Work out the finished part from the listing and answer in its coordinate system (mm). A direction names the side the tool comes from. Give positions to 0.01 mm unless a question says otherwise; leave off trailing zeros. Loops run counter-clockwise (first coordinate to the right, second up) from the corner with the lowest first, then second, coordinate; pieces in that order, holes last. Notation, with made-up numbers: M 6.5,50.5 L 20.5,50.5 A21 cw 20.5,86.5 Z; hole C 51,66 d10. An arc over 180 degrees is marked long. Answer in a Markdown table with one row per item. Add a question column.
from build123d import *

# Parameters (mm, degrees)
F0_R         = 38.1
F0_R_2       = 31.75
F1_DEPTH     = 26.924
F2_R         = 2.4528409794
F4_START     = -34.036
F3_W         = 36.8709713221
F3_H         = 33.7369362824
F4_DEPTH     = 4.826
F5_R         = 5.08
F6_W         = 26.7109713221
F6_H         = 23.5769362824
F7_DEPTH     = 4.826
F8_T1_DEPTH  = 26.7109713221
F8_T3_DEPTH  = 23.5769362824
F8_T6_ANGLE  = 90
F8_T8_ANGLE  = 90
F8_T10_ANGLE = 90
F8_T12_ANGLE = 90
F9_W         = 6.8778875601
F9_H         = 2.9623268638
F10_DEPTH    = 4.8006
F12_START    = 31.75
F11_W        = 2.54
F11_H        = 2.54
F12_DEPTH    = 7.874


# Not quite as in the source:
# - a fillet or chamfer that OpenCascade refuses, or shapes differently, is made with other operations: its cross-section is extruded or revolved along the edge and cut away or added


with BuildPart() as f1:
    # F0 (on Front) → F1 (new body)
    with BuildSketch(Plane.XZ):
        Circle(F0_R)
        Circle(F0_R_2, mode=Mode.SUBTRACT)
    extrude(amount=F1_DEPTH)

    # F2
    f2_edges = [f1.edges().sort_by_distance(p)[0] for p in [
        (-38.1, -26.924, 0),
        (-38.1, 0, 0),
    ]]
    fillet(f2_edges, radius=F2_R)

    # F3 (on Top) → F4 (join)
    with BuildSketch(Plane.XY.offset(F4_START)):
        with Locations((0.0921785831, -14.0109679196)):
            Rectangle(F3_W, F3_H)
    extrude(amount=-F4_DEPTH)

    # F5
    f5_edges = [f1.edges().sort_by_distance(p)[0] for p in [
        (-18.343307, 2.8575, -36.449),
        (18.527664, 2.8575, -36.449),
        (18.527664, -30.879436, -36.449),
        (-18.343307, -30.879436, -36.449),
    ]]
    fillet(f5_edges, radius=F5_R)

    # F6 (on face) → F7 (cut)
    with BuildSketch(Plane(origin=(0, 0, -38.862), x_dir=(1, 0, 0), z_dir=(0, 0, -1))):
        with Locations((0.0921785831, 14.0109679196)):
            Rectangle(F6_W, F6_H)
    extrude(amount=-F7_DEPTH, mode=Mode.SUBTRACT)

    # F8: fillet of radius 5.08 on 1 edges, made by hand

    # F8_s2 → F8_t1 (cut)
    with BuildSketch(Plane.YZ.offset(-13.2633070779)):
        with BuildLine():
            ThreePointArc((-30.8794360608, -34.036), (-29.3069384175, -37.4628096935), (-25.8057900345, -38.862))
            Line((-25.8057900345, -38.862), (-30.8794360608, -38.862))
            Line((-30.8794360608, -38.862), (-30.8794360608, -34.036))
        make_face()
        with BuildLine():
            ThreePointArc((2.8575002216, -34.036), (1.2850025783, -37.4628096935), (-2.2161458047, -38.862))
            Line((-2.2161458047, -38.862), (2.8575002216, -38.862))
            Line((2.8575002216, -38.862), (2.8575002216, -34.036))
        make_face()
    extrude(amount=F8_T1_DEPTH, mode=Mode.SUBTRACT)

    # F8_s4 → F8_t3 (cut)
    with BuildSketch(Plane.XZ.offset(2.2224997784)):
        with BuildLine():
            ThreePointArc((18.5276642442, -34.036), (16.9551666009, -37.4628096935), (13.4540182179, -38.862))
            Line((13.4540182179, -38.862), (18.5276642442, -38.862))
            Line((18.5276642442, -38.862), (18.5276642442, -34.036))
        make_face()
        with BuildLine():
            ThreePointArc((-18.3433070779, -34.036), (-16.7708094346, -37.4628096935), (-13.2696610516, -38.862))
            Line((-13.2696610516, -38.862), (-18.3433070779, -38.862))
            Line((-18.3433070779, -38.862), (-18.3433070779, -34.036))
        make_face()
    extrude(amount=F8_T3_DEPTH, mode=Mode.SUBTRACT)

    # F8_s5 → F8_t6 (revolve, cut)
    with BuildSketch(Plane.YZ.offset(-13.2633070779)):
        with BuildLine():
            ThreePointArc((-30.8794360608, -34.036), (-29.3069384175, -37.4628096935), (-25.8057900345, -38.862))
            Line((-25.8057900345, -38.862), (-30.8794360608, -38.862))
            Line((-30.8794360608, -38.862), (-30.8794360608, -34.036))
        make_face()
    revolve(axis=Axis((-13.2633070779, -25.7994360608, -38.862), (0, 0, -1)), revolution_arc=F8_T6_ANGLE, mode=Mode.SUBTRACT)

    # F8_s7 → F8_t8 (revolve, cut)
    with BuildSketch(Plane.XZ.offset(25.7994360608)):
        with BuildLine():
            ThreePointArc((18.5276642442, -34.036), (16.9551666009, -37.4628096935), (13.4540182179, -38.862))
            Line((13.4540182179, -38.862), (18.5276642442, -38.862))
            Line((18.5276642442, -38.862), (18.5276642442, -34.036))
        make_face()
    revolve(axis=Axis((13.4476642442, -25.7994360608, -38.862), (0, 0, -1)), revolution_arc=F8_T8_ANGLE, mode=Mode.SUBTRACT)

    # F8_s9 → F8_t10 (revolve, cut)
    with BuildSketch(Plane.XZ.offset(2.2224997784)):
        with BuildLine():
            ThreePointArc((18.5276642442, -34.036), (16.9551666009, -37.4628096935), (13.4540182179, -38.862))
            Line((13.4540182179, -38.862), (18.5276642442, -38.862))
            Line((18.5276642442, -38.862), (18.5276642442, -34.036))
        make_face()
    revolve(axis=Axis((13.4476642442, -2.2224997784, -38.862), (0, 0, 1)), revolution_arc=F8_T10_ANGLE, mode=Mode.SUBTRACT)

    # F8_s11 → F8_t12 (revolve, cut)
    with BuildSketch(Plane.YZ.offset(-13.2633070779)):
        with BuildLine():
            ThreePointArc((2.8575002216, -34.036), (1.2850025783, -37.4628096935), (-2.2161458047, -38.862))
            Line((-2.2161458047, -38.862), (2.8575002216, -38.862))
            Line((2.8575002216, -38.862), (2.8575002216, -34.036))
        make_face()
    revolve(axis=Axis((-13.2633070779, -2.2224997784, -38.862), (0, 0, 1)), revolution_arc=F8_T12_ANGLE, mode=Mode.SUBTRACT)

    # F9 (on face) → F10 (join)
    with BuildSketch(Plane(origin=(0, 0, -34.036), x_dir=(1, 0, 0), z_dir=(0, 0, -1))):
        with Locations((-9.8243632978, 12.5298044877)):
            Rectangle(F9_W, F9_H)
    extrude(amount=F10_DEPTH)

    # F11 (on Top) → F12 (join)
    with BuildSketch(Plane.XY.offset(F12_START)):
        with Locations((-0.3243902236, -14.0109681524)):
            Rectangle(F11_W, F11_H)
    extrude(amount=F12_DEPTH)


solid = f1.part
(1) Each of these flat-tipped pins is pushed along its axis until it touches: P1, Ø1.2, axis at x = 0, z = 38.5, coming from the -Y side; P2, Ø1, axis at y = -1, z = -8, coming from the -X side; P3, Ø4, axis at x = -20, y = -8, coming from the +Z side. Where does it stop, or does it pass through?
(2) Which of the six approach directions +Z, -Z, +X, -X, +Y, -Y give full straight-line access (tool end or side, diameter ignored) to faces 4 (the face through (-10, -14.011, -36)), 5 (the face through (16.99, -13.85, -37.43)), 6 (the face through (0, 0, 32))?
(3) Section A-A, the plane z = 0 is taken. Determine the outline of the cut face in (x, y), and give its area (3 significant figures).
(4) Consider line 1 along Z through (x, y) = (-1, -12); line 2 along X through (y, z) = (-18.5, 4); line 3 along X through (y, z) = (-16.5, 25.5). Determine where each line is inside the solid, lowest interval first. Write a range as from..to.
(5) The mould has two halves that part along Z. Classify faces 1 (the face through (-16.81, -13.846, -37.425)), 2 (the face through (-10, -11.049, -36)), 3 (the face through (0, -28, -34.036)): pulls with the +Z half, pulls with the -Z half, needs draft (parallel to the pull), parting line crosses it, or undercut.
Numbers:
| question | item | result |
|---|---|---|
| 1 | P1 | stops at y = -25.44 |
| 1 | P2 | stops at x = -37.08 |
| 1 | P3 | stops at z = 33.58 |
| 2 | face 4 | -Z |
| 2 | face 5 | -Z, +X, +Y, -Y |
| 2 | face 6 | +Z, +X, -X, +Y |
| 3 | outline | M -38.1,-24.47 A2.45 ccw -35.65,-26.92 L -31.75,-26.92 L -31.75,0 L -35.65,0 A2.45 ccw -38.1,-2.45 Z; M 31.75,-26.92 L 35.65,-26.92 A2.45 ccw 38.1,-24.47 L 38.1,-2.45 A2.45 ccw 35.65,0 L 31.75,0 Z |
| 3 | area | 337 mm² |
| 4 | line 1 | z = -34.04..-31.73, 31.73..38.09 |
| 4 | line 2 | x = -37.89..-31.5, 31.5..37.89 |
| 4 | line 3 | x = -28.31..-18.92, 18.92..28.31 |
| 5 | face 1 | pulls with the -Z half |
| 5 | face 2 | needs draft |
| 5 | face 3 | undercut |
